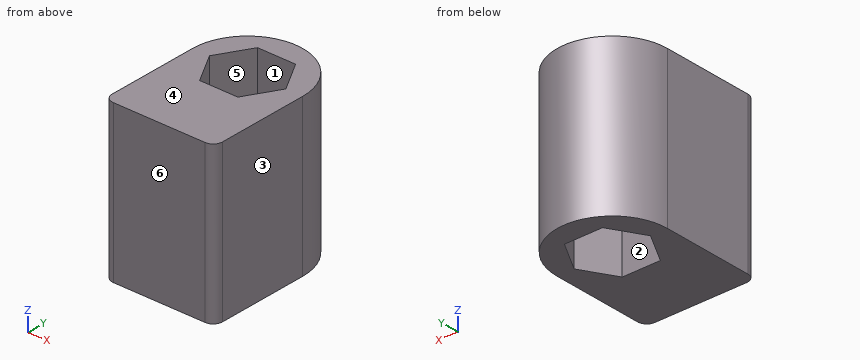
```python
from build123d import *

# Parameters (mm, degrees)
BOSS_EXTRUDE1_DEPTH = 17


with BuildPart() as part:
    # Sketch1 → Boss-Extrude1 (new body)
    with BuildSketch(Plane.XY):
        with BuildLine():
            Line((1, 0), (11, 0))
            ThreePointArc((11, 0), (11.707106781, 0.292893219), (12, 1))
            Line((12, 1), (12, 11))
            ThreePointArc((12, 11), (6, 17), (0, 11))
            Line((0, 11), (0, 1))
            ThreePointArc((0, 1), (0.292893219, 0.292893219), (1, 0))
        make_face()
        Polygon((10.156921938, 11), (8.078460969, 14.6), (3.921539031, 14.6), (1.843078062, 11), (3.921539031, 7.4), (8.078460969, 7.4), align=None, mode=Mode.SUBTRACT)
    extrude(amount=BOSS_EXTRUDE1_DEPTH)


solid = part.part
```
Build history of the part. All positions in model axes, mm. Face numbers are marked on the shaded views. A direction names the side the tool comes from. Coordinates: 2 decimals unless noted, no trailing zeros. Order: outer loops, then holes, each group sorted by start corner. A loop starts at its lowest first (then second) coordinate and runs counter-clockwise, first axis right, second up. Notation, with made-up numbers: M 77,-26.75 L 96,-26.75 A25 cw 96,-3.75 Z; hole C 25.25,-26 d9. An arc over 180 degrees is marked long. One line per question, with ' | ' between items. Start each with the question number.
1. Cut at A-A (x = 6). Write the cut outline in (y, z), plus the area to 3 significant figures.
2. Cut at B-B (y = 8.25). Write the cut outline in (x, z).
3. Cut at D-D (x = 11.25). Write the cut outline in (y, z).
4. Flat gauge pins, fed straight in: P1, Ø1.5, axis at x = 7.5, z = 13.5, coming from the +Y side; P2, Ø1, axis at x = 2.5, y = 11, coming from the +Z side; P3, Ø3, axis at x = 9, z = 6, coming from the +Y side. Where does each tip first touch, or does it go through?
5. Cut at C-C (z = 10). Write the cut outline in (x, y).
6. Mould opens along X. For the marked faces 1, 2, 3 and 4 say: +X half, -X half, draft (parallel to the pull), parting line (faces both ways), or undercut.
7. Tool access for the marked faces 5 and 6: list every direction of +Z, -Z, +X, -X, +Y, -Y with a clear straight run to the whole face (end or side of a thin tool).
8. Wall check: line 1 along Y through (x, z) = (6, 3); line 2 along Y through (x, z) = (3.25, 7.5); line 3 along X through (y, z) = (7.75, 13.5). Give the ranges that are in metal, low to high. Write a range as [from, to].
The answers:
1) outline: M 0,0 L 7.4,0 L 7.4,17 L 0,17 Z; M 14.6,0 L 17,0 L 17,17 L 14.6,17 Z | area: 167 mm2
2) outline: M 0,0 L 3.43,0 L 3.43,17 L 0,17 Z; M 8.57,0 L 12,0 L 12,17 L 8.57,17 Z
3) outline: M 0.03,0 L 13.9,0 L 13.9,17 L 0.03,17 Z
4) P1: stops at y = 16.95 | P2: passes through | P3: stops at y = 16.81
5) outline: M 0,1 A1 ccw 1,0 L 11,0 A1 ccw 12,1 L 12,11 A6 ccw 0,11 Z; hole M 1.84,11 L 3.92,7.4 L 8.08,7.4 L 10.16,11 L 8.08,14.6 L 3.92,14.6 Z
6) face 1: undercut | face 2: undercut | face 3: +X half | face 4: draft
7) face 5: +Z, -Z | face 6: +Z, -Z, +X, -X, -Y
8) line 1: y = [0, 7.4], [14.6, 17] | line 2: y = [0, 8.56], [13.44, 16.33] | line 3: x = [0, 3.72], [8.28, 12]
